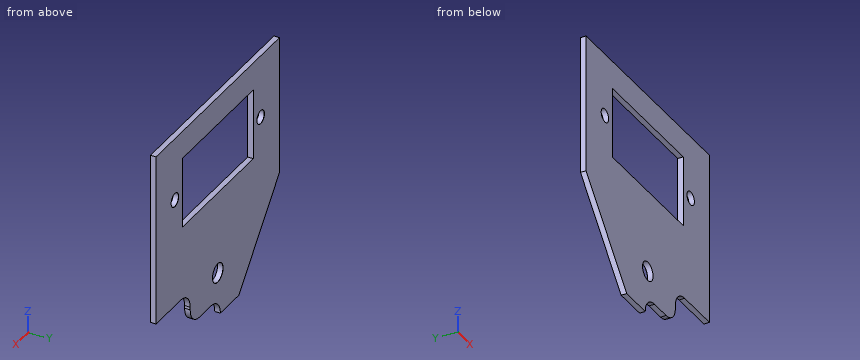
```python
from build123d import *

# Parameters (mm, degrees)
BOSS_EXTRUDE1_DEPTH           = 1
SKETCH4_W                     = 40
SKETCH4_H                     = 25
BOSS_EXTRUDE2_DEPTH           = 1
SKETCH5_W                     = 8.058679656
SKETCH5_H                     = 6
BOSS_EXTRUDE3_DEPTH           = 1
SKETCH8_W                     = 23
SKETCH8_H                     = 12.75
CUT_EXTRUDE1_DEPTH            = 1
M2_CLEARANCE_HOLE1_AT_2_COUNT = 2
M2_CLEARANCE_HOLE1_AT_2_PITCH = 27.8


with BuildPart() as part:
    # Sketch1 → Boss-Extrude1 (new body)
    with BuildSketch(Plane(origin=(0, 0, 0), x_dir=(1, 0, 0), z_dir=(0, 1, 0))):
        with BuildLine():
            Line((-3, 0), (-9, 0))
            Line((-9, 0), (-9, -15.5))
            Line((-9, -15.5), (9.77, -15.5))
            Line((9.77, -15.5), (9.77, -9.5))
            ThreePointArc((9.77, -9.5), (7.648679656, -8.621320344), (6.77, -6.5))
            Line((6.77, -6.5), (6.77, -6))
            ThreePointArc((6.77, -6), (5.891320344, -3.878679656), (3.77, -3))
            Line((3.77, -3), (0, -3))
            ThreePointArc((0, -3), (-2.121320344, -2.121320344), (-3, 0))
        make_face()
    extrude(amount=BOSS_EXTRUDE1_DEPTH)

    # Sketch3 → M3 Clearance Hole1 (revolve, cut)
    with BuildSketch(Plane(origin=(-2.171320344, 1, 7.921320344), x_dir=(0, 0, 1), z_dir=(1, 0, 0))):
        Polygon((0, 0), (0, 1), (1.7, 1), (1.7, 0.025), (1.725, 0), align=None)
    revolve(axis=Axis((-2.171320344, 7.35, 7.921320344), (0, -1, 0)), mode=Mode.SUBTRACT)

    # Sketch4 → Boss-Extrude2 (add)
    with BuildSketch(Plane(origin=(0, 1, 0), x_dir=(1, 0, 0), z_dir=(0, 1, 0))):
        with Locations((-2.171320344, -28)):
            Rectangle(SKETCH4_W, SKETCH4_H)
    extrude(amount=-BOSS_EXTRUDE2_DEPTH)

    # Sketch5 → Boss-Extrude3 (add)
    with BuildSketch(Plane(origin=(0, 1, 0), x_dir=(1, 0, 0), z_dir=(0, 1, 0))):
        with Locations((13.799339828, -12.5)):
            Rectangle(SKETCH5_W, SKETCH5_H)
        Polygon((-9, -15.5), (-22.171320344, -15.5), (-9, 0), align=None)
    extrude(amount=-BOSS_EXTRUDE3_DEPTH)

    # Sketch8 → Cut-Extrude1 (cut)
    with BuildSketch(Plane(origin=(0, 1, 0), x_dir=(1, 0, 0), z_dir=(0, 1, 0))):
        with Locations((-2.171320344, -29.125)):
            Rectangle(SKETCH8_W, SKETCH8_H)
    extrude(amount=-CUT_EXTRUDE1_DEPTH, mode=Mode.SUBTRACT)

    # Sketch10 → M2 Clearance Hole1 (revolve, cut)
    with BuildSketch(Plane(origin=(-16.071320344, 1, 29.125), x_dir=(0, 0, 1), z_dir=(1, 0, 0))):
        Polygon((0, 0), (0, 1), (1.2, 1), (1.2, 0.025), (1.225, 0), align=None)
    m2_clearance_hole1 = revolve(axis=Axis((-16.071320344, 7.35, 29.125), (0, -1, 0)), mode=Mode.SUBTRACT)

    # M2 Clearance Hole1 at 2: M2 Clearance Hole1 ×2
    with Locations(*[(i * M2_CLEARANCE_HOLE1_AT_2_PITCH, 0, 0) for i in range(1, M2_CLEARANCE_HOLE1_AT_2_COUNT)]):
        add(m2_clearance_hole1, mode=Mode.SUBTRACT)


solid = part.part
```
Model file for the job. Use its own axes, mm. Give positions to 0.01 mm unless a question says otherwise; leave off trailing zeros. Loops run counter-clockwise (first coordinate to the right, second up) from the corner with the lowest first, then second, coordinate; pieces in that order, holes last. Notation, with made-up numbers: (73, -30.75) - (132, -30.75) arc R5 ccw to (132, -26.75) - close; hole circle Ø10 at (77.25, 75). An arc over 180 degrees is marked (long way). One line per item, written item: value. Start each with the question number.
1. Slice it at B-B (z = 25). List the corners of the cut face in (x, y), plus the area to 3 significant figures.
2. Slice it at A-A (x = -6). List the corners of the cut face in (y, z).
3. Pin check, flat tip, straight feed: pin 1 (1.4 mm diameter, centred on x = 11.73, z = 29.12, fed in from +Y). Stop position of the tip, or through.
4. Slice it at C-C (y = 0.2). List the corners of the cut face in (x, z) (3 decimals), plus the area to 3 significant figures.
5. Slice it at D-D (x = 14.5). List the corners of the cut face in (y, z).
6. Probe L1, parallel to Z at x = 4, y = 0.5; L2, parallel to Z at x = -8, y = 0.4; L3, parallel to X at y = 0.6, z = 27.5. List the from-to ranges inside material, lowest first. Write a range as from..to.
Solution:
1. outline: (-22.17, 0) - (-13.67, 0) - (-13.67, 1) - (-22.17, 1) - close; (9.33, 0) - (17.83, 0) - (17.83, 1) - (9.33, 1) - close
1. area: 17.0 mm^2
2. outline: (0, 0) - (1, 0) - (1, 22.75) - (0, 22.75) - close; (0, 35.5) - (1, 35.5) - (1, 40.5) - (0, 40.5) - close
3. pin 1: passes through
4. outline: (-22.171, 15.5) - (-9, 0) - (-3, 0) arc R3 cw to (0, 3) - (3.77, 3) arc R3 ccw to (6.77, 6) - (6.77, 6.5) arc R3 cw to (9.77, 9.5) - (17.829, 9.5) - (17.829, 40.5) - (-22.171, 40.5) - close; hole circle Ø2.4 at (-16.071, 29.125); hole (-13.671, 22.75) - (9.329, 22.75) - (9.329, 35.5) - (-13.671, 35.5) - close; hole circle Ø3.4 at (-2.171, 7.921); hole circle Ø2.4 at (11.729, 29.125)
4. area: 1,070 mm^2
5. outline: (0, 9.5) - (1, 9.5) - (1, 40.5) - (0, 40.5) - close
6. L1: z = 3.01..22.75, 35.5..40.5
6. L2: z = 0..22.75, 35.5..40.5
6. L3: x = -22.17..-13.67, 9.33..17.83
